Read the model definition and answer for the solid it produces. Units are mm, in the model's axes. Face numbers are marked on the shaded views. A direction names the side the tool comes from. Round coordinates to 2 decimals unless told otherwise and drop trailing zeros. Order: outer loops, then holes, each group sorted by start corner. A loop starts at its lowest first (then second) coordinate and runs counter-clockwise, first axis right, second up. Notation, with made-up numbers: (49.5, 86.5) - (66.5, 86.5) arc R25 ccw to (66.5, 102.5) - close; hole circle Ø6 at (82, -28.5). An arc over 180 degrees is marked (long way). Answer as a JSON object with one key per item and string values. Group by question number.
Q1. The mould has two halves that part along Z. Classify the marked faces 1, 2 and 3: pulls with the +Z half, pulls with the -Z half, needs draft (parallel to the pull), parting line crosses it, or undercut.
Q2. Consider line 1 (Y direction, x = -23.05, z = 1.15); line 2 (Y direction, x = 22.75, z = 1.9); line 3 (Z direction, x = -6, y = 3.5). Determine where each line is inside the solid, lowest interval first.
Q3. A cutting plane is placed at A-A on z = 3.5. Count the separate pieces of the cut face and the enclosed holes in it, and give its area (3 significant figures).
Q4. A cutting plane is placed at C-C on x = 2.5. Determine the outline of the cut face in (y, z), and give its area (3 significant figures).
Q5. A cutting plane is placed at B-B on y = -11. Determine the outline of the cut face in (x, z).
Q6. A tool of negligible diameter and unlimited length cuts with its end or side. For the marked faces 4, 5 and 6, from which of +Z, -Z, +X, -X, +Y, -Y can it reach the whole face along a straight path? Write none if from no direction.
Q7. A cutting plane is placed at D-D on y = 4. Determine the outline of the cut face in (x, z), and give its area (3 significant figures).
Q8. Given pin 1 Ø6 at (x, y) = (-15, -16) entering from +Z; pin 2 Ø1.5 at (x, y) = (13, 10) entering from -Z; pin 3 Ø2.5 at (x, y) = (0, 6.477) entering from -Z; pin 4 Ø0.7 at (x, y) = (7, 0) entering from -Z, each flat-ended and moving along its own axis, determine where each tip first touches the part or whether it passes through.
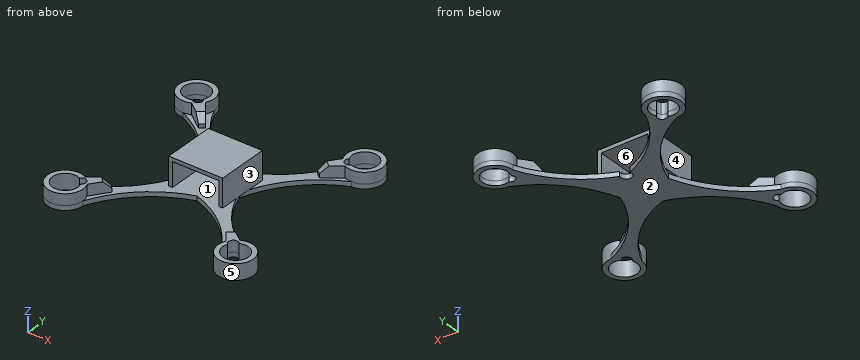
```python
from build123d import *
from build123d import SkipClean  # not in build123d's __all__

# Parameters (mm, degrees)
F0_R     = 3.45
F1_DEPTH = 1.25
F2_R     = 1.27
F3_DEPTH = 15.24
F5_DEPTH = 7
F6_R     = 1.5
F7_DEPTH = 1.25
F9_DEPTH = 3
F10_SIZE = 2


# Not quite as in the source:
# - a feature of the source that left no trace in its solid (it failed there, or was rolled back) is left out


with BuildPart() as f1:
    # F0 (on Top) → F1 (new body)
    with BuildSketch(Plane.XY):
        with BuildLine():
            ThreePointArc((0, 6.477), (-10.7423411653, 12.8214445823), (-17.975, 22.987))
            ThreePointArc((-17.975, 22.987), (-26.1154007446, 26.3744330736), (-22.7811582525, 18.2121016594))
            ThreePointArc((-22.7811582525, 18.2121016594), (-12.6900771407, 10.8419183213), (-6.477, 0))
            ThreePointArc((-6.477, 0), (-12.7950799481, -10.8797937043), (-23.0188417475, -18.2121016594))
            ThreePointArc((-23.0188417475, -18.2121016594), (-26.4374330736, -26.3524007446), (-18.275, -22.987))
            ThreePointArc((-18.275, -22.987), (-10.9098200432, -12.770210249), (0, -6.477))
            ThreePointArc((0, -6.477), (10.9098200432, -12.770210249), (18.275, -22.987))
            ThreePointArc((18.275, -22.987), (26.4374330736, -26.3524007446), (23.0188417475, -18.2121016594))
            ThreePointArc((23.0188417475, -18.2121016594), (12.7950799481, -10.8797937043), (6.477, 0))
            ThreePointArc((6.477, 0), (12.6900771407, 10.8419183213), (22.7811582525, 18.2121016594))
            ThreePointArc((22.7811582525, 18.2121016594), (26.1154007446, 26.3744330736), (17.975, 22.987))
            ThreePointArc((17.975, 22.987), (10.7423411653, 12.8214445823), (0, 6.477))
        make_face()
        with Locations((-23.05, -22.987)):
            Circle(F0_R, mode=Mode.SUBTRACT)
        with Locations((23.05, -22.987)):
            Circle(F0_R, mode=Mode.SUBTRACT)
        with Locations((-22.75, 22.987)):
            Circle(F0_R, mode=Mode.SUBTRACT)
        with Locations((22.75, 22.987)):
            Circle(F0_R, mode=Mode.SUBTRACT)
    extrude(amount=F1_DEPTH)

    # F2 (on face) → F3 (cut)
    with BuildSketch(Plane.XY.offset(1.25)):
        with Locations((-20.5791849834, 20.5791849834)):
            Circle(F2_R)
        with Locations((20.5791849834, 20.5791849834)):
            Circle(F2_R)
        with Locations((20.5791849834, -20.5791849834)):
            Circle(F2_R)
        with Locations((-20.5791849834, -20.5791849834)):
            Circle(F2_R)
    extrude(amount=-F3_DEPTH, mode=Mode.SUBTRACT)

    # F4 (on Front) → F5 (join, symmetric)
    with BuildSketch(Plane.XZ):
        Polygon((-6.3, 1.25), (-6.3, 7.85), (6.3, 7.85), (6.3, 1.25), (7.3, 1.25), (7.3, 8.85), (-7.3, 8.85), (-7.3, 1.25), align=None)
    extrude(amount=F5_DEPTH, both=True)

    # F6 (on face) → F7 (cut, through all)
    with BuildSketch(Plane.XY.offset(1.25)):
        with Locations((0, 6.477)):
            Circle(F6_R)
    extrude(amount=-F7_DEPTH, mode=Mode.SUBTRACT)

    # F8 (on face) → F9 (join)
    with BuildSketch(Plane.XY.offset(1.25)):
        with BuildLine():
            Line((-16.3602319323, -15.5348950992), (-20.8478584952, -18.7501146118))
            ThreePointArc((-20.8478584952, -18.7501146118), (-26.4716233511, -26.3176333696), (-18.7553139698, -20.8998256177))
            Line((-18.7553139698, -20.8998256177), (-15.5117037948, -16.3834232366))
            Line((-15.5117037948, -16.3834232366), (-16.3602319323, -15.5348950992))
        make_face()
        with BuildLine():
            ThreePointArc((-19.8753821862, -21.6363328551), (-25.5208150166, -25.3948150166), (-21.6178063096, -19.8483185518))
            ThreePointArc((-21.6178063096, -19.8483185518), (-19.669638586, -19.6928298904), (-19.8753821862, -21.6363328551))
        make_face(mode=Mode.SUBTRACT)
        with BuildLine():
            Line((15.3199540065, -16.3082468694), (18.7838269987, -20.8421473423))
            ThreePointArc((18.7838269987, -20.8421473423), (26.4264348802, -26.3634348802), (20.9051473423, -18.7208269987))
            Line((20.9051473423, -18.7208269987), (16.5119000472, -15.3976071843))
            Line((16.5119000472, -15.3976071843), (15.3199540065, -16.3082468694))
        make_face()
        with BuildLine():
            ThreePointArc((21.6178063096, -19.8483185518), (25.5208150166, -25.3948150166), (19.8753821862, -21.6363328551))
            ThreePointArc((19.8753821862, -21.6363328551), (19.669638586, -19.6928298904), (21.6178063096, -19.8483185518))
        make_face(mode=Mode.SUBTRACT)
        with BuildLine():
            Line((16.3457305073, 15.2946304795), (20.7653185529, 18.6439982094))
            ThreePointArc((20.7653185529, 18.6439982094), (25.9985065626, 26.4866900024), (18.5665604362, 20.6849447408))
            Line((18.5665604362, 20.6849447408), (15.1525434236, 16.2036434514))
            Line((15.1525434236, 16.2036434514), (16.3457305073, 15.2946304795))
        make_face()
        with BuildLine():
            ThreePointArc((19.659038987, 21.4545313979), (25.0601507831, 25.5493628469), (21.5448562878, 19.7543341291))
            ThreePointArc((21.5448562878, 19.7543341291), (19.7287816517, 19.6359383702), (19.659038987, 21.4545313979))
        make_face(mode=Mode.SUBTRACT)
        with BuildLine():
            ThreePointArc((-18.5665604362, 20.6849447408), (-25.9985065626, 26.4866900024), (-20.7653185529, 18.6439982094))
            Line((-20.7653185529, 18.6439982094), (-16.3523570468, 15.30128828))
            Line((-16.3523570468, 15.30128828), (-15.1589701598, 16.2100389266))
            Line((-15.1589701598, 16.2100389266), (-18.5665604362, 20.6849447408))
        make_face()
        with BuildLine():
            ThreePointArc((-21.5448562878, 19.7543341291), (-25.0601507831, 25.5493628469), (-19.659038987, 21.4545313979))
            ThreePointArc((-19.659038987, 21.4545313979), (-19.3094528761, 20.6052689951), (-19.6238661036, 19.7423661036))
            ThreePointArc((-19.6238661036, 19.7423661036), (-20.5870970996, 19.30920963), (-21.5448562878, 19.7543341291))
        make_face(mode=Mode.SUBTRACT)
    with SkipClean():  # cleaning this boolean's faces spoils the solid; the shape is the same uncleaned
        extrude(amount=F9_DEPTH)

    # F10
    f10_edges = [f1.edges().sort_by_distance(p)[0] for p in [
        (-15.755664, 15.755664, 4.25),
        (-15.935968, -15.959159, 4.25),
        (15.915927, -15.852927, 4.25),
        (15.749137, 15.749137, 4.25),
    ]]
    chamfer(f10_edges, length=F10_SIZE)


solid = f1.part
```
Result set:
{
 "1": {"face 1": "undercut", "face 2": "pulls with the -Z half", "face 3": "needs draft"},
 "2": {"line 1": "y = -27.76 to -26.44, -19.54 to -18.21, 18.22 to 19.55, 26.42 to 27.75", "line 2": "y = -27.75 to -26.42, -19.55 to -18.22, 18.21 to 19.54, 26.44 to 27.76", "line 3": "z = 0 to 1.25, 7.85 to 8.85"},
 "3": {"separate pieces": "6", "enclosed holes": "4", "area": "194 mm²"},
 "4": {"outline": "(-7.41, 0) - (7.44, 0) - (7.44, 1.25) - (-7.41, 1.25) - close; (-7, 7.85) - (7, 7.85) - (7, 8.85) - (-7, 8.85) - close", "area": "32.6 mm²"},
 "5": {"outline": "(-12.9, 0) - (-8.76, 0) - (-8.76, 1.25) - (-12.9, 1.25) - close; (8.76, 0) - (12.9, 0) - (12.9, 1.25) - (8.76, 1.25) - close"},
 "6": {"face 4": "+Z, -X, +Y, -Y", "face 5": "+Z", "face 6": "+Y, -Y"},
 "7": {"outline": "(-8.09, 0) - (8.09, 0) - (8.09, 1.25) - (7.3, 1.25) - (7.3, 8.85) - (-7.3, 8.85) - (-7.3, 1.25) - (-8.09, 1.25) - close; hole (-6.3, 1.25) - (6.3, 1.25) - (6.3, 7.85) - (-6.3, 7.85) - close", "area": "48.0 mm²"},
 "8": {"pin 1": "stops at z = 4.25", "pin 2": "passes through", "pin 3": "stops at z = 7.85", "pin 4": "stops at z = 1.25"}
}
